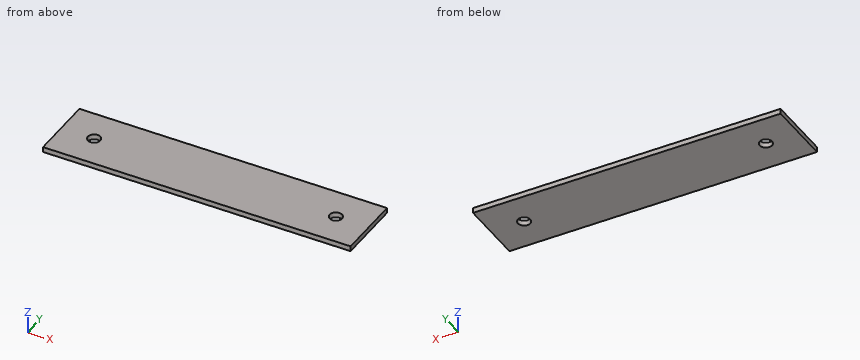
```python
from build123d import *

# Parameters (mm, degrees)
SKETCH1_W             = 93.54
SKETCH1_H             = 20
BOSS_EXTRUDE1_DEPTH   = 1.5875
F_6_CLEARANCE_HOLE1_D = 3.7973


with BuildPart() as part:
    # Sketch1 → Boss-Extrude1 (new body)
    with BuildSketch(Plane.XY):
        Rectangle(SKETCH1_W, SKETCH1_H)
    extrude(amount=BOSS_EXTRUDE1_DEPTH)

    # #6 Clearance Hole1 (through all)
    with Locations(Plane.XY.offset(1.5875)):
        with Locations((-36.77, 0), (36.77, 0)):
            Hole(F_6_CLEARANCE_HOLE1_D / 2)


solid = part.part
```
Work out the finished part from the listing and answer in its coordinate system (mm). Give positions to 0.01 mm unless a question says otherwise; leave off trailing zeros. Order: outer loops, then holes, each group sorted by start corner. A loop starts at its lowest first (then second) coordinate and runs counter-clockwise, first axis right, second up.
1. Section A-A, the plane y = 0 is taken. Determine the outline of the cut face in (x, z), and give its area (3 significant figures).
Result sheet:
outline: (-46.77, 0) - (-38.67, 0) - (-38.67, 1.59) - (-46.77, 1.59) - close; (-34.87, 0) - (34.87, 0) - (34.87, 1.59) - (-34.87, 1.59) - close; (38.67, 0) - (46.77, 0) - (46.77, 1.59) - (38.67, 1.59) - close
area: 136 mm2
2. This flat-tipped pin is pushed along its axis until it touches: P1, Ø6, axis at x = -36.77, y = 0, coming from the +Z side. Where does it stop, or does it pass through?
Result sheet:
P1: stops at z = 1.59
3. Straight lines are drawn through the part: L1, parallel to Y at x = -36.77, z = 0.8; L2, parallel to X at y = 0.5, z = 1.2. For each, find the intervals that lie inside material, in ascending order.
Result sheet:
L1: y = -10 to -1.9, 1.9 to 10
L2: x = -46.77 to -38.6, -34.94 to 34.94, 38.6 to 46.77
4. Section B-B, the plane x = -36.77 is taken. Determine the outline of the cut face in (y, z).
Result sheet:
outline: (-10, 0) - (-1.9, 0) - (-1.9, 1.59) - (-10, 1.59) - close; (1.9, 0) - (10, 0) - (10, 1.59) - (1.9, 1.59) - close
